Check sheet for the modelled part. Datum: model origin and axes. Units: mm. Give positions to 0.01 mm unless a question says otherwise; leave off trailing zeros. Loops run counter-clockwise (first coordinate to the right, second up) from the corner with the lowest first, then second, coordinate; pieces in that order, holes last. Notation, with made-up numbers: (86, 12.5) - (98, 12.5) arc R17 ccw to (98, 31.5) - close; hole circle Ø11 at (70, 70.5). An arc over 180 degrees is marked (long way). Answer in a Markdown table with one row per item. Add a question column.
(1) Sectioned sample at A-A on y = -6.3. State how many separate pieces and enclosed holes the cut face has, then the cut area to 3 significant figures.
(2) Sectioned sample at B-B on x = 1.5. Enter the section's corners in (y, z).
(3) Draft check along X on faces 1 (the face through (8.7, -2, 13)), 2 (the face through (-8.207, -3.517, 23.976)), 3 (the face through (-7.7, 0, 10)). Enter one of: released by +X, released by -X, zero draft, split by the parting line, or undercut.
(4) Thickness scan on L1, parallel to Z at x = -8.15, y = 5.7; L2, parallel to X at y = 7.25, z = 11.25; L3, parallel to Y at x = 2.5, z = 6. Record the ranges inside material, lowest first.
from build123d import *

# Parameters (mm, degrees)
EXTRUDE_1_DEPTH                   = 25.5
SKETCH_2_R                        = 1
CUT_EXTRUDE_1_DEPTH               = 27
PATTERN_LINEAR_1_COUNT            = 6
PATTERN_LINEAR_1_PITCH            = 3
PATTERN_LINEAR_2_COUNT            = 6
PATTERN_LINEAR_2_PITCH            = 5
PATTERN_LINEAR_2_COPY_1_SKETCH_R  = 1
PATTERN_LINEAR_2_COPY_1_DEPTH     = 27
PATTERN_LINEAR_2_COPY_2_SKETCH_R  = 1
PATTERN_LINEAR_2_COPY_2_DEPTH     = 27
PATTERN_LINEAR_2_COPY_3_SKETCH_R  = 1
PATTERN_LINEAR_2_COPY_3_DEPTH     = 27
PATTERN_LINEAR_2_COPY_4_SKETCH_R  = 1
PATTERN_LINEAR_2_COPY_4_DEPTH     = 27
PATTERN_LINEAR_2_COPY_5_SKETCH_R  = 1
PATTERN_LINEAR_2_COPY_5_DEPTH     = 27
PATTERN_LINEAR_2_COPY_6_SKETCH_R  = 1
PATTERN_LINEAR_2_COPY_6_DEPTH     = 27
PATTERN_LINEAR_2_COPY_7_SKETCH_R  = 1
PATTERN_LINEAR_2_COPY_7_DEPTH     = 27
PATTERN_LINEAR_2_COPY_8_SKETCH_R  = 1
PATTERN_LINEAR_2_COPY_8_DEPTH     = 27
PATTERN_LINEAR_2_COPY_9_SKETCH_R  = 1
PATTERN_LINEAR_2_COPY_9_DEPTH     = 27
PATTERN_LINEAR_2_COPY_10_SKETCH_R = 1
PATTERN_LINEAR_2_COPY_10_DEPTH    = 27
PATTERN_LINEAR_2_COPY_11_SKETCH_R = 1
PATTERN_LINEAR_2_COPY_11_DEPTH    = 27
PATTERN_LINEAR_2_COPY_12_SKETCH_R = 1
PATTERN_LINEAR_2_COPY_12_DEPTH    = 27
PATTERN_LINEAR_2_COPY_13_SKETCH_R = 1
PATTERN_LINEAR_2_COPY_13_DEPTH    = 27
PATTERN_LINEAR_2_COPY_14_SKETCH_R = 1
PATTERN_LINEAR_2_COPY_14_DEPTH    = 27
PATTERN_LINEAR_2_COPY_15_SKETCH_R = 1
PATTERN_LINEAR_2_COPY_15_DEPTH    = 27
PATTERN_LINEAR_2_COPY_16_SKETCH_R = 1
PATTERN_LINEAR_2_COPY_16_DEPTH    = 27
PATTERN_LINEAR_2_COPY_17_SKETCH_R = 1
PATTERN_LINEAR_2_COPY_17_DEPTH    = 27
PATTERN_LINEAR_2_COPY_18_SKETCH_R = 1
PATTERN_LINEAR_2_COPY_18_DEPTH    = 27
PATTERN_LINEAR_2_COPY_19_SKETCH_R = 1
PATTERN_LINEAR_2_COPY_19_DEPTH    = 27
PATTERN_LINEAR_2_COPY_20_SKETCH_R = 1
PATTERN_LINEAR_2_COPY_20_DEPTH    = 27
PATTERN_LINEAR_2_COPY_21_SKETCH_R = 1
PATTERN_LINEAR_2_COPY_21_DEPTH    = 27
PATTERN_LINEAR_2_COPY_22_SKETCH_R = 1
PATTERN_LINEAR_2_COPY_22_DEPTH    = 27
PATTERN_LINEAR_2_COPY_23_SKETCH_R = 1
PATTERN_LINEAR_2_COPY_23_DEPTH    = 27
PATTERN_LINEAR_2_COPY_24_SKETCH_R = 1
PATTERN_LINEAR_2_COPY_24_DEPTH    = 27
PATTERN_LINEAR_2_COPY_25_SKETCH_R = 1
PATTERN_LINEAR_2_COPY_25_DEPTH    = 27


with BuildPart() as part:
    # 草图1 → 凸台-拉伸1 (new body)
    with BuildSketch(Plane.XY):
        Polygon((-8.7, 10.7), (8.7, 10.7), (8.7, -10.7), (7.7, -10.7), (7.7, 9.7), (-7.7, 9.7), (-7.7, -10.7), (-8.7, -10.7), align=None)
    extrude(amount=EXTRUDE_1_DEPTH)

    # 草图2 → 切除-拉伸1 (cut)
    with BuildSketch(Plane.ZY.offset(8.7)):
        with Locations(Location((3, 8.7, 0), (0, 0, 90))):
            Circle(SKETCH_2_R)
    cut_extrude_1 = extrude(amount=-CUT_EXTRUDE_1_DEPTH, mode=Mode.SUBTRACT)

    # 阵列(线性)1: 切除-拉伸1 ×6
    with Locations(*[(0, -i * PATTERN_LINEAR_1_PITCH, 0) for i in range(1, PATTERN_LINEAR_1_COUNT)]):
        add(cut_extrude_1, mode=Mode.SUBTRACT)

    # 阵列(线性)2: 切除-拉伸1 ×6
    with Locations(*[(0, 0, i * PATTERN_LINEAR_2_PITCH) for i in range(1, PATTERN_LINEAR_2_COUNT)]):
        add(cut_extrude_1, mode=Mode.SUBTRACT)

    # 阵列(线性)2 copy 1 sketch → 阵列(线性)2 copy 1 (cut)
    with BuildSketch(Plane(origin=(-8.7, -3, 5), x_dir=(0, 0, 1), z_dir=(-1, 0, 0))):
        with Locations(Location((3, 8.7, 0), (0, 0, 90))):
            Circle(PATTERN_LINEAR_2_COPY_1_SKETCH_R)
    extrude(amount=-PATTERN_LINEAR_2_COPY_1_DEPTH, mode=Mode.SUBTRACT)

    # 阵列(线性)2 copy 2 sketch → 阵列(线性)2 copy 2 (cut)
    with BuildSketch(Plane(origin=(-8.7, -3, 10), x_dir=(0, 0, 1), z_dir=(-1, 0, 0))):
        with Locations(Location((3, 8.7, 0), (0, 0, 90))):
            Circle(PATTERN_LINEAR_2_COPY_2_SKETCH_R)
    extrude(amount=-PATTERN_LINEAR_2_COPY_2_DEPTH, mode=Mode.SUBTRACT)

    # 阵列(线性)2 copy 3 sketch → 阵列(线性)2 copy 3 (cut)
    with BuildSketch(Plane(origin=(-8.7, -3, 15), x_dir=(0, 0, 1), z_dir=(-1, 0, 0))):
        with Locations(Location((3, 8.7, 0), (0, 0, 90))):
            Circle(PATTERN_LINEAR_2_COPY_3_SKETCH_R)
    extrude(amount=-PATTERN_LINEAR_2_COPY_3_DEPTH, mode=Mode.SUBTRACT)

    # 阵列(线性)2 copy 4 sketch → 阵列(线性)2 copy 4 (cut)
    with BuildSketch(Plane(origin=(-8.7, -3, 20), x_dir=(0, 0, 1), z_dir=(-1, 0, 0))):
        with Locations(Location((3, 8.7, 0), (0, 0, 90))):
            Circle(PATTERN_LINEAR_2_COPY_4_SKETCH_R)
    extrude(amount=-PATTERN_LINEAR_2_COPY_4_DEPTH, mode=Mode.SUBTRACT)

    # 阵列(线性)2 copy 5 sketch → 阵列(线性)2 copy 5 (cut)
    with BuildSketch(Plane(origin=(-8.7, -3, 25), x_dir=(0, 0, 1), z_dir=(-1, 0, 0))):
        with Locations(Location((3, 8.7, 0), (0, 0, 90))):
            Circle(PATTERN_LINEAR_2_COPY_5_SKETCH_R)
    extrude(amount=-PATTERN_LINEAR_2_COPY_5_DEPTH, mode=Mode.SUBTRACT)

    # 阵列(线性)2 copy 6 sketch → 阵列(线性)2 copy 6 (cut)
    with BuildSketch(Plane(origin=(-8.7, -6, 5), x_dir=(0, 0, 1), z_dir=(-1, 0, 0))):
        with Locations(Location((3, 8.7, 0), (0, 0, 90))):
            Circle(PATTERN_LINEAR_2_COPY_6_SKETCH_R)
    extrude(amount=-PATTERN_LINEAR_2_COPY_6_DEPTH, mode=Mode.SUBTRACT)

    # 阵列(线性)2 copy 7 sketch → 阵列(线性)2 copy 7 (cut)
    with BuildSketch(Plane(origin=(-8.7, -6, 10), x_dir=(0, 0, 1), z_dir=(-1, 0, 0))):
        with Locations(Location((3, 8.7, 0), (0, 0, 90))):
            Circle(PATTERN_LINEAR_2_COPY_7_SKETCH_R)
    extrude(amount=-PATTERN_LINEAR_2_COPY_7_DEPTH, mode=Mode.SUBTRACT)

    # 阵列(线性)2 copy 8 sketch → 阵列(线性)2 copy 8 (cut)
    with BuildSketch(Plane(origin=(-8.7, -6, 15), x_dir=(0, 0, 1), z_dir=(-1, 0, 0))):
        with Locations(Location((3, 8.7, 0), (0, 0, 90))):
            Circle(PATTERN_LINEAR_2_COPY_8_SKETCH_R)
    extrude(amount=-PATTERN_LINEAR_2_COPY_8_DEPTH, mode=Mode.SUBTRACT)

    # 阵列(线性)2 copy 9 sketch → 阵列(线性)2 copy 9 (cut)
    with BuildSketch(Plane(origin=(-8.7, -6, 20), x_dir=(0, 0, 1), z_dir=(-1, 0, 0))):
        with Locations(Location((3, 8.7, 0), (0, 0, 90))):
            Circle(PATTERN_LINEAR_2_COPY_9_SKETCH_R)
    extrude(amount=-PATTERN_LINEAR_2_COPY_9_DEPTH, mode=Mode.SUBTRACT)

    # 阵列(线性)2 copy 10 sketch → 阵列(线性)2 copy 10 (cut)
    with BuildSketch(Plane(origin=(-8.7, -6, 25), x_dir=(0, 0, 1), z_dir=(-1, 0, 0))):
        with Locations(Location((3, 8.7, 0), (0, 0, 90))):
            Circle(PATTERN_LINEAR_2_COPY_10_SKETCH_R)
    extrude(amount=-PATTERN_LINEAR_2_COPY_10_DEPTH, mode=Mode.SUBTRACT)

    # 阵列(线性)2 copy 11 sketch → 阵列(线性)2 copy 11 (cut)
    with BuildSketch(Plane(origin=(-8.7, -9, 5), x_dir=(0, 0, 1), z_dir=(-1, 0, 0))):
        with Locations(Location((3, 8.7, 0), (0, 0, 90))):
            Circle(PATTERN_LINEAR_2_COPY_11_SKETCH_R)
    extrude(amount=-PATTERN_LINEAR_2_COPY_11_DEPTH, mode=Mode.SUBTRACT)

    # 阵列(线性)2 copy 12 sketch → 阵列(线性)2 copy 12 (cut)
    with BuildSketch(Plane(origin=(-8.7, -9, 10), x_dir=(0, 0, 1), z_dir=(-1, 0, 0))):
        with Locations(Location((3, 8.7, 0), (0, 0, 90))):
            Circle(PATTERN_LINEAR_2_COPY_12_SKETCH_R)
    extrude(amount=-PATTERN_LINEAR_2_COPY_12_DEPTH, mode=Mode.SUBTRACT)

    # 阵列(线性)2 copy 13 sketch → 阵列(线性)2 copy 13 (cut)
    with BuildSketch(Plane(origin=(-8.7, -9, 15), x_dir=(0, 0, 1), z_dir=(-1, 0, 0))):
        with Locations(Location((3, 8.7, 0), (0, 0, 90))):
            Circle(PATTERN_LINEAR_2_COPY_13_SKETCH_R)
    extrude(amount=-PATTERN_LINEAR_2_COPY_13_DEPTH, mode=Mode.SUBTRACT)

    # 阵列(线性)2 copy 14 sketch → 阵列(线性)2 copy 14 (cut)
    with BuildSketch(Plane(origin=(-8.7, -9, 20), x_dir=(0, 0, 1), z_dir=(-1, 0, 0))):
        with Locations(Location((3, 8.7, 0), (0, 0, 90))):
            Circle(PATTERN_LINEAR_2_COPY_14_SKETCH_R)
    extrude(amount=-PATTERN_LINEAR_2_COPY_14_DEPTH, mode=Mode.SUBTRACT)

    # 阵列(线性)2 copy 15 sketch → 阵列(线性)2 copy 15 (cut)
    with BuildSketch(Plane(origin=(-8.7, -9, 25), x_dir=(0, 0, 1), z_dir=(-1, 0, 0))):
        with Locations(Location((3, 8.7, 0), (0, 0, 90))):
            Circle(PATTERN_LINEAR_2_COPY_15_SKETCH_R)
    extrude(amount=-PATTERN_LINEAR_2_COPY_15_DEPTH, mode=Mode.SUBTRACT)

    # 阵列(线性)2 copy 16 sketch → 阵列(线性)2 copy 16 (cut)
    with BuildSketch(Plane(origin=(-8.7, -12, 5), x_dir=(0, 0, 1), z_dir=(-1, 0, 0))):
        with Locations(Location((3, 8.7, 0), (0, 0, 90))):
            Circle(PATTERN_LINEAR_2_COPY_16_SKETCH_R)
    extrude(amount=-PATTERN_LINEAR_2_COPY_16_DEPTH, mode=Mode.SUBTRACT)

    # 阵列(线性)2 copy 17 sketch → 阵列(线性)2 copy 17 (cut)
    with BuildSketch(Plane(origin=(-8.7, -12, 10), x_dir=(0, 0, 1), z_dir=(-1, 0, 0))):
        with Locations(Location((3, 8.7, 0), (0, 0, 90))):
            Circle(PATTERN_LINEAR_2_COPY_17_SKETCH_R)
    extrude(amount=-PATTERN_LINEAR_2_COPY_17_DEPTH, mode=Mode.SUBTRACT)

    # 阵列(线性)2 copy 18 sketch → 阵列(线性)2 copy 18 (cut)
    with BuildSketch(Plane(origin=(-8.7, -12, 15), x_dir=(0, 0, 1), z_dir=(-1, 0, 0))):
        with Locations(Location((3, 8.7, 0), (0, 0, 90))):
            Circle(PATTERN_LINEAR_2_COPY_18_SKETCH_R)
    extrude(amount=-PATTERN_LINEAR_2_COPY_18_DEPTH, mode=Mode.SUBTRACT)

    # 阵列(线性)2 copy 19 sketch → 阵列(线性)2 copy 19 (cut)
    with BuildSketch(Plane(origin=(-8.7, -12, 20), x_dir=(0, 0, 1), z_dir=(-1, 0, 0))):
        with Locations(Location((3, 8.7, 0), (0, 0, 90))):
            Circle(PATTERN_LINEAR_2_COPY_19_SKETCH_R)
    extrude(amount=-PATTERN_LINEAR_2_COPY_19_DEPTH, mode=Mode.SUBTRACT)

    # 阵列(线性)2 copy 20 sketch → 阵列(线性)2 copy 20 (cut)
    with BuildSketch(Plane(origin=(-8.7, -12, 25), x_dir=(0, 0, 1), z_dir=(-1, 0, 0))):
        with Locations(Location((3, 8.7, 0), (0, 0, 90))):
            Circle(PATTERN_LINEAR_2_COPY_20_SKETCH_R)
    extrude(amount=-PATTERN_LINEAR_2_COPY_20_DEPTH, mode=Mode.SUBTRACT)

    # 阵列(线性)2 copy 21 sketch → 阵列(线性)2 copy 21 (cut)
    with BuildSketch(Plane(origin=(-8.7, -15, 5), x_dir=(0, 0, 1), z_dir=(-1, 0, 0))):
        with Locations(Location((3, 8.7, 0), (0, 0, 90))):
            Circle(PATTERN_LINEAR_2_COPY_21_SKETCH_R)
    extrude(amount=-PATTERN_LINEAR_2_COPY_21_DEPTH, mode=Mode.SUBTRACT)

    # 阵列(线性)2 copy 22 sketch → 阵列(线性)2 copy 22 (cut)
    with BuildSketch(Plane(origin=(-8.7, -15, 10), x_dir=(0, 0, 1), z_dir=(-1, 0, 0))):
        with Locations(Location((3, 8.7, 0), (0, 0, 90))):
            Circle(PATTERN_LINEAR_2_COPY_22_SKETCH_R)
    extrude(amount=-PATTERN_LINEAR_2_COPY_22_DEPTH, mode=Mode.SUBTRACT)

    # 阵列(线性)2 copy 23 sketch → 阵列(线性)2 copy 23 (cut)
    with BuildSketch(Plane(origin=(-8.7, -15, 15), x_dir=(0, 0, 1), z_dir=(-1, 0, 0))):
        with Locations(Location((3, 8.7, 0), (0, 0, 90))):
            Circle(PATTERN_LINEAR_2_COPY_23_SKETCH_R)
    extrude(amount=-PATTERN_LINEAR_2_COPY_23_DEPTH, mode=Mode.SUBTRACT)

    # 阵列(线性)2 copy 24 sketch → 阵列(线性)2 copy 24 (cut)
    with BuildSketch(Plane(origin=(-8.7, -15, 20), x_dir=(0, 0, 1), z_dir=(-1, 0, 0))):
        with Locations(Location((3, 8.7, 0), (0, 0, 90))):
            Circle(PATTERN_LINEAR_2_COPY_24_SKETCH_R)
    extrude(amount=-PATTERN_LINEAR_2_COPY_24_DEPTH, mode=Mode.SUBTRACT)

    # 阵列(线性)2 copy 25 sketch → 阵列(线性)2 copy 25 (cut)
    with BuildSketch(Plane(origin=(-8.7, -15, 25), x_dir=(0, 0, 1), z_dir=(-1, 0, 0))):
        with Locations(Location((3, 8.7, 0), (0, 0, 90))):
            Circle(PATTERN_LINEAR_2_COPY_25_SKETCH_R)
    extrude(amount=-PATTERN_LINEAR_2_COPY_25_DEPTH, mode=Mode.SUBTRACT)


solid = part.part
Reply:
| question | item | result |
|---|---|---|
| 1 | separate pieces | 12 |
| 1 | enclosed holes | 0 |
| 1 | area | 31.0 mm^2 |
| 2 | outline | (9.7, 0) - (10.7, 0) - (10.7, 25.5) - (9.7, 25.5) - close |
| 3 | face 1 | released by +X |
| 3 | face 2 | zero draft |
| 3 | face 3 | undercut |
| 4 | L1 | 0 to 2, 4 to 7, 9 to 12, 14 to 17, 19 to 22, 24 to 25.5 |
| 4 | L2 | -8.7 to -7.7, 7.7 to 8.7 |
| 4 | L3 | 9.7 to 10.7 |
